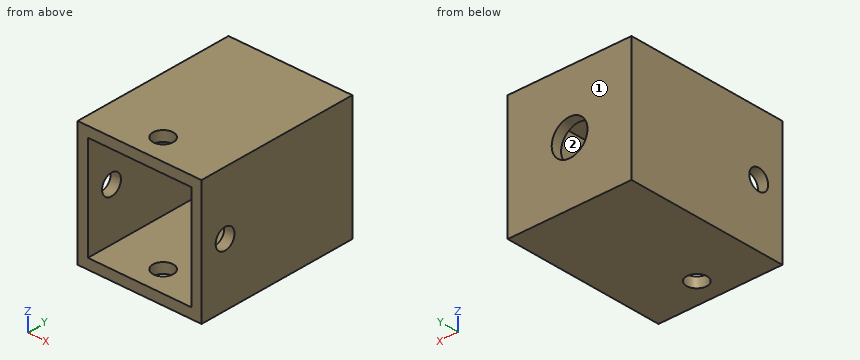
```python
from build123d import *

# Parameters (mm, degrees)
SKETCH1_W           = 24.2
SKETCH1_H           = 24.2
SKETCH1_W_2         = 20.2
SKETCH1_H_2         = 20.2
BOSS_EXTRUDE1_DEPTH = 30
SKETCH2_R           = 2
CUT_EXTRUDE1_DEPTH  = 30
SKETCH3_R           = 2
CUT_EXTRUDE2_DEPTH  = 30
SKETCH4_W           = 24.2
SKETCH4_H           = 24.2
SKETCH4_R           = 3.5
BOSS_EXTRUDE2_DEPTH = 2


with BuildPart() as part:
    # Sketch1 → Boss-Extrude1 (new body)
    with BuildSketch(Plane(origin=(0, 0, 0), x_dir=(1, 0, 0), z_dir=(0, 1, 0))):
        Rectangle(SKETCH1_W, SKETCH1_H)
        Rectangle(SKETCH1_W_2, SKETCH1_H_2, mode=Mode.SUBTRACT)
    extrude(amount=BOSS_EXTRUDE1_DEPTH)

    # Sketch2 → Cut-Extrude1 (cut)
    with BuildSketch(Plane.XY.offset(12.1)):
        with Locations((0, 5)):
            Circle(SKETCH2_R)
    extrude(amount=-CUT_EXTRUDE1_DEPTH, mode=Mode.SUBTRACT)

    # Sketch3 → Cut-Extrude2 (cut)
    with BuildSketch(Plane(origin=(12.1, 0, 0), x_dir=(0, 0, -1), z_dir=(1, 0, 0))):
        with Locations((0, 5)):
            Circle(SKETCH3_R)
    extrude(amount=-CUT_EXTRUDE2_DEPTH, mode=Mode.SUBTRACT)

    # Sketch4 → Boss-Extrude2 (add)
    with BuildSketch(Plane(origin=(0, 30, 0), x_dir=(1, 0, 0), z_dir=(0, 1, 0))):
        Rectangle(SKETCH4_W, SKETCH4_H)
        with Locations(Location((0, 0, 0), (0, 0, 270))):
            Circle(SKETCH4_R, mode=Mode.SUBTRACT)
    extrude(amount=BOSS_EXTRUDE2_DEPTH)


solid = part.part
```
The listing builds one solid part. Answer for the finished solid, in the listing's coordinates (mm). Face numbers are marked on the shaded views. A direction names the side the tool comes from. Give positions to 0.01 mm unless a question says otherwise; leave off trailing zeros. Order: outer loops, then holes, each group sorted by start corner. A loop starts at its lowest first (then second) coordinate and runs counter-clockwise, first axis right, second up. Notation, with made-up numbers: M -9.75,78 L 12.25,78 A24 cw 12.25,101 Z; hole C 63.25,3 d9. An arc over 180 degrees is marked long. Put each result on its own line as item: value. Start each with the question number.
Item 1: The part is cut by section A-A, the plane x = 0. Determine the outline of the cut face in (y, z).
Item 2: Which of the six approach directions +Z, -Z, +X, -X, +Y, -Y give full straight-line access (tool end or side, diameter ignored) to the marked faces 1 and 2?
Item 3: The part is cut by section B-B, the plane z = 0. Determine the outline of the cut face in (x, y).
Item 4: Find the intervals of material crossed by line 1 along X through (y, z) = (5, -5.5); line 2 along Y through (x, z) = (0, 10.9), in increasing order.
Item 5: The part is cut by section D-D, the plane y = 5. Determine the outline of the cut face in (x, z), and give its area (3 significant figures).
Item 6: The part is cut by section C-C, the plane y = 14.5. Determine the outline of the cut face in (x, z).
Item 7: A flat-ended cylindrical pin translates along its axis: P1, Ø6, axis at x = -0.5, z = 2.5, coming from the -Y side. Find the tip coordinate at first contact, or state that the pin passes through.
Answer key:
1. outline: M 0,-12.1 L 3,-12.1 L 3,-10.1 L 0,-10.1 Z; M 0,10.1 L 3,10.1 L 3,12.1 L 0,12.1 Z; M 7,-12.1 L 32,-12.1 L 32,-3.5 L 30,-3.5 L 30,-10.1 L 7,-10.1 Z; M 7,10.1 L 30,10.1 L 30,3.5 L 32,3.5 L 32,12.1 L 7,12.1 Z
2. face 1: +Z, -Z, +X, -X, +Y
2. face 2: -Y
3. outline: M -12.1,0 L -10.1,0 L -10.1,3 L -12.1,3 Z; M -12.1,7 L -10.1,7 L -10.1,30 L -3.5,30 L -3.5,32 L -12.1,32 Z; M 3.5,30 L 10.1,30 L 10.1,7 L 12.1,7 L 12.1,32 L 3.5,32 Z; M 10.1,0 L 12.1,0 L 12.1,3 L 10.1,3 Z
4. line 1: x = -12.1 to -10.1, 10.1 to 12.1
4. line 2: y = 0 to 3, 7 to 32
5. outline: M -12.1,-12.1 L -2,-12.1 L -2,-10.1 L -10.1,-10.1 L -10.1,-2 L -12.1,-2 Z; M -12.1,2 L -10.1,2 L -10.1,10.1 L -2,10.1 L -2,12.1 L -12.1,12.1 Z; M 2,-12.1 L 12.1,-12.1 L 12.1,-2 L 10.1,-2 L 10.1,-10.1 L 2,-10.1 Z; M 2,10.1 L 10.1,10.1 L 10.1,2 L 12.1,2 L 12.1,12.1 L 2,12.1 Z
5. area: 146 mm²
6. outline: M -12.1,-12.1 L 12.1,-12.1 L 12.1,12.1 L -12.1,12.1 Z; hole M -10.1,-10.1 L 10.1,-10.1 L 10.1,10.1 L -10.1,10.1 Z
7. P1: stops at y = 30
